For this review, use the dimensioned drawing (mm, ordinates from the lowest corner) and the shaded views. Coordinates: 2 decimals unless noted, no trailing zeros. Loops run counter-clockwise (first coordinate to the right, second up) from the corner with the lowest first, then second, coordinate; pieces in that order, holes last.
1. Clearance check with flat-ended pins moving along their axes: P1, Ø1.5, axis at x = 150, z = 1.5, coming from the -Y side; P2, Ø16, axis at x = 40, y = 30, coming from the -Z side; P3, Ø1.5, axis at y = 58.5, z = 2, coming from the -X side; P4, Ø0.9, axis at y = 31, z = 1.5, coming from the +X side. State where each tip first meets the part, or that it passes through.
2. Take a section at B-B, the plane z = 0.95. Count the separate pieces of the cut face and the enclosed holes in it, then the cut area to 3 significant figures.
3. To check wall thickness, follow probe 1 along X at (y, z) = (30.5, 2.35); probe 2 along X at (y, z) = (26.5, 0.95); probe 3 along Y at (x, z) = (68, 0.95). State the ranges of each line that lie inside material, in increasing order.
4. Take a section at A-A, the plane y = 30. State the section outline as (x, z) points, then the cut area to 3 significant figures.
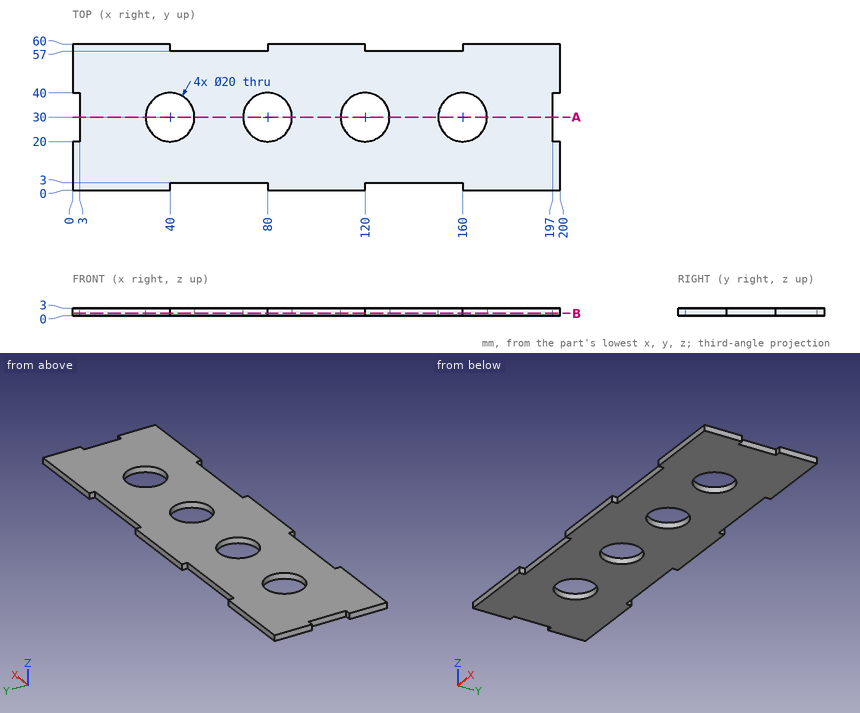
Results list:
1. P1: stops at y = 3
1. P2: passes through
1. P3: stops at x = 0
1. P4: stops at x = 197
2. separate pieces: 1
2. enclosed holes: 4
2. area: 10,100 mm2
3. probe 1: x = 3 to 30.01, 49.99 to 70.01, 89.99 to 110.01, 129.99 to 150.01, 169.99 to 197
3. probe 2: x = 3 to 30.63, 49.37 to 70.63, 89.37 to 110.63, 129.37 to 150.63, 169.37 to 197
3. probe 3: y = 3 to 57
4. outline: (3, 0) - (30, 0) - (30, 3) - (3, 3) - close; (50, 0) - (70, 0) - (70, 3) - (50, 3) - close; (90, 0) - (110, 0) - (110, 3) - (90, 3) - close; (130, 0) - (150, 0) - (150, 3) - (130, 3) - close; (170, 0) - (197, 0) - (197, 3) - (170, 3) - close
4. area: 342 mm2
